Here's how the part is built. I have some questions about the finished solid (model axes, mm). A direction names the side the tool comes from. Coordinates: 2 decimals unless noted, no trailing zeros. Loops run counter-clockwise (first coordinate to the right, second up) from the corner with the lowest first, then second, coordinate; pieces in that order, holes last. Notation, with made-up numbers: (-22.75, 16.5) -> (-17.75, 16.5) arc R25 ccw to (-17.75, 45.5) -> close; hole circle Ø10 at (77, -18.5). An arc over 180 degrees is marked (long way). Answer as a JSON object with one key per item and string values. Group by question number.
Q1. I want a section at A-A on x = -6. Write out the boundary of the cut face in (y, z).
Q2. I'm going to push flat-ended pins straight in: pin 1 (3 mm diameter, centred on x = -7.5, y = -21.5, fed in from -Z); pin 2 (1 mm diameter, centred on x = 22.5, z = 5.5, fed in from -Y); pin 3 (3 mm diameter, centred on x = 27.5, z = 5, fed in from -Y); pin 4 (3 mm diameter, centred on x = 6.5, z = 3, fed in from -Y). Where does each tip first touch, or does it pass through?
Q3. I want a section at D-D on x = 9. Write out the boundary of the cut face in (y, z).
Q4. I want a section at B-B on y = -61. Write out the boundary of the cut face in (x, z), then the cut area to 3 significant figures.
Q5. Thinking about a two-plate mould opening in Y: for faces 1 (the flat face through (13, -22, 10)), 2 (the flat face through (7, -5.279, 5)), 3 (the flat face through (-1, -20.279, 5)), which applies, released by +Y, released by -Y, zero draft, split by the parting line, or undercut?
Q6. On a 3-axis mill with a long thin cutter (end or side, diameter ignored), from which of +Z, -Z, +X, -X, +Y, -Y can I reach the whole of each face in a straight line? I mean faces 4 (the cylindrical face through (2, -48, 5)), 5 (the cylindrical face through (24.2, -17.7, 5.1)), 6 (the flat face through (1.608, -50, 5)), 7 (the flat face through (-23.392, -15, 5)). Say none if no direction works.
Q7. I need wall thicknesses on line 1 (X direction, y = -14.5, z = 3); line 2 (X direction, y = -21.5, z = 5.5); line 3 (Y direction, x = -9, z = 4.75). Which ranges of each line are inside material? Lowest first, please.
```python
from build123d import *

# Parameters (mm, degrees)
F0_W     = 8
F0_H     = 8
F1_DEPTH = 10
F2_R     = 2
F3_R     = 17.49999
F4_R     = 2.49999


# Not quite as in the source:
# - a fillet or chamfer is up to 0.001 mm smaller than in the source, because OpenCascade refuses the exact size
# - a feature names something its author has since deleted; it is built from what else it names


with BuildPart() as f1:
    # F0 (on Top) → F1 (new body)
    with BuildSketch(Plane.XY):
        Polygon((-18.3916796818, -10.2785023413), (-23.3916796818, -10.2785023413), (-23.3916796818, -25.2785023413), (21.6083203182, -25.2785023413), (21.6083203182, -18.2785023413), (21.6083203182, -10.2785023413), (16.6083203182, -10.2785023413), (16.6083203182, -20.2785023413), (-18.3916796818, -20.2785023413), align=None)
        Polygon((-23.3916796818, -5.2785023413), (-23.3916796818, -10.2785023413), (-18.3916796818, -10.2785023413), (16.6083203182, -10.2785023413), (21.6083203182, -10.2785023413), (23.6083203182, -10.2785023413), (31.6083203182, -10.2785023413), (36.6083203182, -10.2785023413), (36.6083203182, -5.2785023413), align=None)
        with Locations((27.6083203182, -14.2785023413)):
            Rectangle(F0_W, F0_H)
        Polygon((36.6083203182, -36.2785023413), (36.6083203182, -10.2785023413), (31.6083203182, -10.2785023413), (31.6083203182, -18.2785023413), (31.6083203182, -36.2785023413), align=None)
        with BuildLine():
            Line((36.6083203182, -68.7785023413), (36.6083203182, -36.2785023413))
            Line((36.6083203182, -36.2785023413), (31.6083203182, -36.2785023413))
            Line((31.6083203182, -36.2785023413), (31.6083203182, -46.8433834612))
            Line((31.6083203182, -46.8433834612), (31.6083203182, -51.2785023413))
            ThreePointArc((31.6083203182, -51.2785023413), (19.1083203182, -63.7785023413), (6.6083203182, -51.2785023413))
            Line((6.6083203182, -51.2785023413), (6.6083203182, -46.8433834612))
            Line((6.6083203182, -46.8433834612), (1.6083203182, -46.8433834612))
            Line((1.6083203182, -46.8433834612), (1.6083203182, -68.7785023413))
            Line((1.6083203182, -68.7785023413), (36.6083203182, -68.7785023413))
        make_face()
    extrude(amount=F1_DEPTH)

    # F2
    f2_edges = [f1.edges().sort_by_distance(p)[0] for p in [
        (-23.39168, -25.278502, 5),
        (21.60832, -25.278502, 5),
        (23.60832, -18.278502, 5),
        (36.60832, -5.278502, 5),
        (-23.39168, -5.278502, 5),
    ]]
    fillet(f2_edges, radius=F2_R)

    # F3 (radius 17.5 in the source; OpenCascade refuses exactly that, so slightly less here)
    f3_edges = [f1.edges().sort_by_distance(p)[0] for p in [
        (1.60832, -68.778502, 5),
        (36.60832, -68.778502, 5),
    ]]
    fillet(f3_edges, radius=F3_R)

    # F4 (radius 2.5 in the source; OpenCascade refuses exactly that, so slightly less here)
    f4_edges = [f1.edges().sort_by_distance(p)[0] for p in [
        (1.60832, -46.843383, 5),
        (6.60832, -46.843383, 5),
        (-18.39168, -20.278502, 5),
        (-18.39168, -10.278502, 5),
        (16.60832, -10.278502, 5),
        (16.60832, -20.278502, 5),
    ]]
    fillet(f4_edges, radius=F4_R)


solid = f1.part
```
Result set:
{
 "1": {"outline": "(-25.28, 0) -> (-20.28, 0) -> (-20.28, 10) -> (-25.28, 10) -> close; (-10.28, 0) -> (-5.28, 0) -> (-5.28, 10) -> (-10.28, 10) -> close"},
 "2": {"pin 1": "stops at z = 0", "pin 2": "stops at y = -68.54", "pin 3": "stops at y = -67.36", "pin 4": "stops at y = -64.8"},
 "3": {"outline": "(-65.56, 0) -> (-58.63, 0) -> (-58.63, 10) -> (-65.56, 10) -> close; (-25.28, 0) -> (-20.28, 0) -> (-20.28, 10) -> (-25.28, 10) -> close; (-10.28, 0) -> (-5.28, 0) -> (-5.28, 10) -> (-10.28, 10) -> close"},
 "4": {"outline": "(4.56, 0) -> (11.25, 0) -> (11.25, 10) -> (4.56, 10) -> close; (26.97, 0) -> (33.66, 0) -> (33.66, 10) -> (26.97, 10) -> close", "area": "134 mm²"},
 "5": {"face 1": "zero draft", "face 2": "released by +Y", "face 3": "undercut"},
 "6": {"face 4": "+Z, -Z, -X", "face 5": "+Z, -Z", "face 6": "+Z, -Z, -X, -Y", "face 7": "+Z, -Z, -X, +Y, -Y"},
 "7": {"line 1": "x = -23.39 to -18.39, 16.61 to 21.61, 23.61 to 36.61", "line 2": "x = -23.39 to 21.61, 31.61 to 36.61", "line 3": "y = -25.28 to -20.28, -10.28 to -5.28"}
}
